from build123d import *

# Parameters (mm, degrees)
F0_W      = 100
F0_H      = 200
F1_DEPTH  = 20
F3_DEPTH  = 10
F5_DEPTH  = 20
F6_R      = 45
F6_R_2    = 30
F7_DEPTH  = 10
F8_R      = 30
F9_DEPTH  = 22
F10_R     = 5
F11_DEPTH = 25


with BuildPart() as f1:
    # F0 (on Front) → F1 (new body)
    with BuildSketch(Plane.XZ):
        with Locations((50, -100)):
            Rectangle(F0_W, F0_H)
    extrude(amount=F1_DEPTH)

    # F2 (on face) → F3 (cut)
    with BuildSketch(Plane(origin=(0, 0, 0), x_dir=(-1, 0, 0), z_dir=(0, 1, 0))):
        with BuildLine():
            ThreePointArc((-90, -178), (-86.485281, -186.485281), (-78, -190))
            Line((-78, -190), (-22, -190))
            ThreePointArc((-22, -190), (-13.514719, -186.485281), (-10, -178))
            Line((-10, -178), (-10, -172))
            ThreePointArc((-10, -172), (-13.514719, -163.514719), (-22, -160))
            Line((-22, -160), (-78, -160))
            ThreePointArc((-78, -160), (-86.485281, -163.514719), (-90, -172))
            Line((-90, -172), (-90, -178))
        make_face()
    extrude(amount=-F3_DEPTH, mode=Mode.SUBTRACT)

    # F4 (on face) → F5 (join)
    with BuildSketch(Plane(origin=(0, 0, 0), x_dir=(-1, 0, 0), z_dir=(0, 1, 0))):
        with BuildLine():
            Line((-89, -148), (-11, -148))
            ThreePointArc((-11, -148), (-3.928932, -145.071068), (-1, -138))
            Line((-1, -138), (-1, -65.448764))
            ThreePointArc((-1, -65.448764), (-1.676281, -61.477192), (-3.628897, -57.95327))
            Line((-3.628897, -57.95327), (-39.39, -13.243608))
            ThreePointArc((-39.39, -13.243608), (-52.117284, -8.319647), (-63.566855, -15.745039))
            Line((-63.566855, -15.745039), (-96.467366, -57.988184))
            ThreePointArc((-96.467366, -57.988184), (-98.349194, -61.463537), (-99, -65.361716))
            Line((-99, -65.361716), (-99, -138))
            ThreePointArc((-99, -138), (-96.071068, -145.071068), (-89, -148))
        make_face()
    extrude(amount=F5_DEPTH)

    # F6 (on face) → F7 (join)
    with BuildSketch(Plane(origin=(0, 20, 0), x_dir=(-1, 0, 0), z_dir=(0, 1, 0))):
        with Locations((-50, -100)):
            Circle(F6_R)
        with Locations((-50, -100)):
            Circle(F6_R_2, mode=Mode.SUBTRACT)
    extrude(amount=F7_DEPTH)

    # F8 (on face) → F9 (cut)
    with BuildSketch(Plane(origin=(0, 20, 0), x_dir=(-1, 0, 0), z_dir=(0, 1, 0))):
        with Locations((-50, -100)):
            Circle(F8_R)
    extrude(amount=-F9_DEPTH, mode=Mode.SUBTRACT)

    # F10 (on face) → F11 (cut)
    with BuildSketch(Plane(origin=(0, 30, 0), x_dir=(-1, 0, 0), z_dir=(0, 1, 0))):
        with Locations((-87.5, -100)):
            Circle(F10_R)
        with Locations((-12.5, -100)):
            Circle(F10_R)
        with Locations((-50, -137.5)):
            Circle(F10_R)
        with Locations((-50, -62.5)):
            Circle(F10_R)
    extrude(amount=-F11_DEPTH, mode=Mode.SUBTRACT)


solid = f1.part
Geometry check sheet. Reference: the model listing, model coordinates, mm. A direction names the side the tool comes from. Give positions to 0.01 mm unless a question says otherwise; leave off trailing zeros. Loops run counter-clockwise (first coordinate to the right, second up) from the corner with the lowest first, then second, coordinate; pieces in that order, holes last. Notation, with made-up numbers: (29.25, 65) -> (41.25, 65) arc R36 ccw to (41.25, 99) -> close; hole circle Ø10 at (33, 21). An arc over 180 degrees is marked (long way). Answer in a Markdown table with one row per item. Add a question column.
1) Cross-section at A-A on y = 27.5. Record the boundary of the cut face in (x, z), and give its area (3 significant figures).
2) Set-up check for faces 4 (the face through (1.66, 9.86, -61.53)), 5 (the face through (51, 10, -148)), 6 (the face through (50, -5, -190)): record each of +Z, -Z, +X, -X, +Y, -Y from which the full face is reachable in a straight line by a thin tool's end or side.
3) Draft check along Z on faces 1 (the face through (51.9, 9.9, -8.3)), 2 (the face through (99, 10, -101)), 3 (the face through (50, 5, -62)). Enter one of: pulls with the +Z half, pulls with the -Z half, needs draft (parallel to the pull), parting line crosses it, or undercut.
4) Material ranges on probe 1 along Z at (x, y) = (50, 14.25); probe 2 along Y at (x, z) = (55.5, -127); probe 3 along X at (y, z) = (16, -62), recorded low to high. Write a range as from..to.
5) Cross-section at D-D on x = 59.5. Record the boundary of the cut face in (y, z).
6) Cross-section at B-B on x = 26.5. Record the boundary of the cut face in (y, z), and give its area (3 significant figures).
7) Gauge pin test, flat ends, axial feed: P1, Ø11.5, axis at x = 87.5, z = -100, coming from the +Y side; P2, Ø1, axis at x = 88.5, y = 16, coming from the +Z side; P3, Ø3, axis at x = 48.5, z = -135.5, coming from the +Y side; P4, Ø10, axis at y = 15, z = -107, coming from the -X side. Record the tip position at first contact, or that the pin passes through.
8) Cross-section at C-C on z = -62.5. Record the boundary of the cut face in (x, y), and give its area (3 significant figures).
Outcome:
| question | item | result |
|---|---|---|
| 1 | outline | circle Ø90 at (50, -100); hole circle Ø10 at (12.5, -100); hole circle Ø60 at (50, -100); hole circle Ø10 at (50, -137.5); hole circle Ø10 at (50, -62.5); hole circle Ø10 at (87.5, -100) |
| 1 | area | 3,220 mm^2 |
| 2 | face 4 | +Z, -X, +Y |
| 2 | face 5 | -Z, +X, -X, +Y |
| 2 | face 6 | +Y |
| 3 | face 1 | pulls with the +Z half |
| 3 | face 2 | needs draft |
| 3 | face 3 | undercut |
| 4 | probe 1 | z = -148..-142.5, -132.5..-130, -70..-67.5, -57.5..-8.25 |
| 4 | probe 2 | y = -20..-2 |
| 4 | probe 3 | x = 1.51..45.03, 54.97..98.52 |
| 5 | outline | (-20, -200) -> (0, -200) -> (0, -190) -> (-10, -190) -> (-10, -160) -> (0, -160) -> (0, -148) -> (20, -148) -> (20, -143.99) -> (30, -143.99) -> (30, -128.46) -> (-2, -128.46) -> (-2, -71.54) -> (30, -71.54) -> (30, -56.01) -> (20, -56.01) -> (20, -11.19) -> (0, -11.19) -> (0, 0) -> (-20, 0) -> close |
| 6 | outline | (-20, -200) -> (0, -200) -> (0, -190) -> (-10, -190) -> (-10, -160) -> (0, -160) -> (0, -148) -> (20, -148) -> (20, -138.38) -> (30, -138.38) -> (30, -118.65) -> (-2, -118.65) -> (-2, -81.35) -> (30, -81.35) -> (30, -61.62) -> (20, -61.62) -> (20, -29.36) -> (0, -29.36) -> (0, 0) -> (-20, 0) -> close |
| 6 | area | 5,650 mm^2 |
| 7 | P1 | stops at y = 30 |
| 7 | P2 | stops at z = -47.12 |
| 7 | P3 | stops at y = 5 |
| 7 | P4 | stops at x = 1 |
| 8 | outline | (0, -20) -> (100, -20) -> (100, 0) -> (98.65, 0) -> (98.65, 20) -> (74.87, 20) -> (74.87, 30) -> (55, 30) -> (55, 5) -> (45, 5) -> (45, 30) -> (25.13, 30) -> (25.13, 20) -> (1.37, 20) -> (1.37, 0) -> (0, 0) -> close |
| 8 | area | 4,190 mm^2 |
